from build123d import *

# Parameters (mm, degrees)
SKETCH1_R                = 3
BOSS_EXTRUDE1_DEPTH      = 5
BOSS_EXTRUDE2_DEPTH      = 5
BOSS_EXTRUDE2_DEPTH_BACK = 9
SKETCH2_R                = 2


with BuildPart() as part:
    # Sketch1 → Boss-Extrude1 (new body)
    with BuildSketch(Plane(origin=(0, 0, 0), x_dir=(0, 0, -1), z_dir=(1, 0, 0))):
        Circle(SKETCH1_R)
    extrude(amount=BOSS_EXTRUDE1_DEPTH)

    # Sketch2 → Boss-Extrude2 (add, two sides: drawn at the far end of the back side and taken through both)
    with BuildSketch(Plane(origin=(5, 0, 0), x_dir=(0, 0, -1), z_dir=(1, 0, 0)).offset(-BOSS_EXTRUDE2_DEPTH_BACK)):
        Circle(SKETCH2_R)
    extrude(amount=BOSS_EXTRUDE2_DEPTH + BOSS_EXTRUDE2_DEPTH_BACK)


solid = part.part
Geometry check sheet. Reference: the model listing, model coordinates, mm. A direction names the side the tool comes from. Round coordinates to 2 decimals unless told otherwise and drop trailing zeros. Write each loop counter-clockwise with the first axis right and the second up, starting at its lowest first coordinate (ties: lowest second). Pieces come first, ordered by that corner, then holes.
Item 1: Section check D-D (x = 2). Record the boundary of the cut face in (y, z).
Determined:
outline: circle Ø6 at (0, 0)
Item 2: Go/stop test with a flat-tipped pin: pin 1 Ø3 at (x, z) = (-2, 2.5) entering from -Y. Record where the tip stops, or that it passes through.
Determined:
pin 1: stops at y = -1.73
Item 3: Material ranges on line 1 along X through (y, z) = (1.4, -2.3); line 2 along Y through (x, z) = (4.75, 0.15); line 3 along Y through (x, z) = (1, -2.55), recorded low to high.
Determined:
line 1: x = 0 to 5
line 2: y = -3 to 3
line 3: y = -1.58 to 1.58
Item 4: Section check C-C (x = -2.5). Record the boundary of the cut face in (y, z), plus the area to 3 significant figures.
Determined:
outline: circle Ø4 at (0, 0)
area: 12.6 mm2
Item 5: Access from +Z, -Z, +X, -X, +Y, -Y to the whole of each face (thin tool, end or side, straight path). Record for faces 1 (the face through (-2, -2, 0)), 2 (the face through (10, 0, 0)), 3 (the face through (5, -2, -1)).
Determined:
face 1: -X
face 2: +Z, -Z, +X, +Y, -Y
face 3: +X
Item 6: Section check A-A (y = 0). Record the boundary of the cut face in (x, z).
Determined:
outline: (-4, -2) - (0, -2) - (0, -3) - (5, -3) - (5, -2) - (10, -2) - (10, 2) - (5, 2) - (5, 3) - (0, 3) - (0, 2) - (-4, 2) - close
